```python
from build123d import *

# Parameters (mm, degrees)
SKETCH1_W                = 95.885
SKETCH1_H                = 90.17
SKETCH1_R                = 3.175
BOSS_EXTRUDE1_DEPTH      = 25.4
BOSS_EXTRUDE2_DEPTH      = 28.575
BOSS_EXTRUDE2_DEPTH_BACK = 3.175
SKETCH1_2_R              = 3.175


with BuildPart() as part:
    # Sketch1 → Boss-Extrude1 (new body)
    with BuildSketch(Plane(origin=(0, 0, 0), x_dir=(1, 0, 0), z_dir=(0, 1, 0))):
        Rectangle(SKETCH1_W, SKETCH1_H)
        with Locations(Location((-42.8625, 37.465, 0), (0, 0, 270))):
            Circle(SKETCH1_R, mode=Mode.SUBTRACT)
        with Locations(Location((-42.8625, -36.195, 0), (0, 0, 270))):
            Circle(SKETCH1_R, mode=Mode.SUBTRACT)
        with Locations(Location((42.8625, 40.005, 0), (0, 0, 270))):
            Circle(SKETCH1_R, mode=Mode.SUBTRACT)
        with Locations(Location((42.8625, -40.005, 0), (0, 0, 270))):
            Circle(SKETCH1_R, mode=Mode.SUBTRACT)
    extrude(amount=BOSS_EXTRUDE1_DEPTH)

    # Sketch1_2 → Boss-Extrude2 (add, two sides: drawn at the far end of the back side and taken through both)
    with BuildSketch(Plane(origin=(0, 0, 0), x_dir=(1, 0, 0), z_dir=(0, 1, 0)).offset(-BOSS_EXTRUDE2_DEPTH_BACK)):
        with Locations(Location((-42.8625, -36.195, 0), (0, 0, 270))):
            Circle(SKETCH1_2_R)
        with Locations(Location((-42.8625, 37.465, 0), (0, 0, 270))):
            Circle(SKETCH1_2_R)
        with Locations(Location((42.8625, 40.005, 0), (0, 0, 270))):
            Circle(SKETCH1_2_R)
        with Locations(Location((42.8625, -40.005, 0), (0, 0, 270))):
            Circle(SKETCH1_2_R)
    extrude(amount=BOSS_EXTRUDE2_DEPTH + BOSS_EXTRUDE2_DEPTH_BACK)


solid = part.part
```
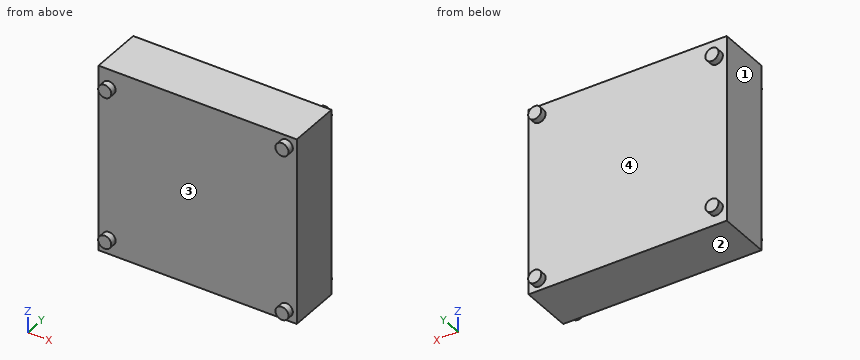
Geometry check sheet. Reference: the model listing, model coordinates, mm. Face numbers are marked on the shaded views. Round coordinates to 2 decimals unless told otherwise and drop trailing zeros. Order: outer loops, then holes, each group sorted by start corner. A loop starts at its lowest first (then second) coordinate and runs counter-clockwise, first axis right, second up. Notation, with made-up numbers: (-11, -28.75) - (39, -28.75) arc R17 ccw to (39, -10.75) - close; hole circle Ø7 at (33, 77.5). An arc over 180 degrees is marked (long way). Use a Markdown table: item, result. Add a question column.
(1) Material ranges on line 1 along Y through (x, z) = (16, 11), recorded low to high. Write a range as [from, to].
(2) Sectioned sample at C-C, the plane x = -8. Enter the section's corners in (y, z) (3 decimals), and give its area (3 significant figures).
(3) Depth check by flat-ended pin: pin 1 (12 mm diameter, centred on x = -37, z = -24, fed in from -Y); pin 2 (1 mm diameter, centred on x = -32, z = 30, fed in from +Y). Enter the tip coordinate at first touch or a pass-through.
(4) Sectioned sample at B-B, the plane z = 15. Enter the section's corners in (x, y), and give its area (3 significant figures).
(5) Release check for a two-part mould opening along Z. For the marked faces 1, 2, 3 and 4 record: pulls with the +Z half, pulls with the -Z half, needs draft (parallel to the pull), parting line crosses it, or undercut.
(6) Sectioned sample at A-A, the plane x = 41. Enter the section's corners in (y, z) (3 decimals), and give its area (3 significant figures).
Answers below:
| question | item | result |
|---|---|---|
| 1 | line 1 | [0, 25.4] |
| 2 | outline | (0, -45.085) - (25.4, -45.085) - (25.4, 45.085) - (0, 45.085) - close |
| 2 | area | 2,290 mm² |
| 3 | pin 1 | y = 0 |
| 3 | pin 2 | y = 25.4 |
| 4 | outline | (-47.94, 0) - (47.94, 0) - (47.94, 25.4) - (-47.94, 25.4) - close |
| 4 | area | 2,440 mm² |
| 5 | face 1 | needs draft |
| 5 | face 2 | pulls with the -Z half |
| 5 | face 3 | undercut |
| 5 | face 4 | undercut |
| 6 | outline | (-3.175, -42.576) - (0, -42.576) - (0, -45.085) - (25.4, -45.085) - (25.4, -42.576) - (28.575, -42.576) - (28.575, -37.434) - (25.4, -37.434) - (25.4, 37.434) - (28.575, 37.434) - (28.575, 42.576) - (25.4, 42.576) - (25.4, 45.085) - (0, 45.085) - (0, 42.576) - (-3.175, 42.576) - (-3.175, 37.434) - (0, 37.434) - (0, -37.434) - (-3.175, -37.434) - close |
| 6 | area | 2,360 mm² |
